Geometry check sheet. Reference: the model listing, model coordinates, mm. A direction names the side the tool comes from. Give positions to 0.01 mm unless a question says otherwise; leave off trailing zeros. Order: outer loops, then holes, each group sorted by start corner. A loop starts at its lowest first (then second) coordinate and runs counter-clockwise, first axis right, second up. Notation, with made-up numbers: M 73.25,65 L 112.25,65 A19 ccw 112.25,77 Z; hole C 32.5,15 d11. An arc over 180 degrees is marked long. Answer as CSV lines item,"result".
Autodesk Inventor part; units mm, degrees
ref_plane "Work Plane1" through (25.25, 10.625, -39.4) normal (1, 0, 0) x (0, 1, 0)
ref_plane "YZ Plane" through (0, 0, 0) normal (1, 0, 0) x (0, 1, 0)
ref_plane "XZ Plane" through (0, 0, 0) normal (0, 1, 0) x (-1, 0, 0)
sketch "Sketch2" plane through (0, 0, 0) normal (0, 1, 0) x (-1, 0, 0)
  line L0 (0, 0) -> (-20, 0)
  line L1 (-20, 0) -> (-20, -66)
  line L2 (-20, -66) -> (0, -66)
  line L3 (0, -66) -> (0, 0)
  dimension "d0" = 20
  dimension "d1" = 66
extrude "Extrusion1" add sketch "Sketch2" along normal blind 30.5
sketch "Sketch3" plane through (20, 0, 0) normal (1, 0, 0) x (0, 0, -1)
  line L0 (39.4, 20.369) -> (34.4, 20.369)
  line L1 (39.4, 10.125) -> (34.4, 10.125)
  line L2 (34.4, 18.9168) -> (34.4, 10.625)
  line L3 (34.4, 20.369) -> (34.4, 18.9308)
  line L4 (0, 0) -> (0, 30.5)
  line L5 (34.4, 20.369) -> (0, 20.369)
  line L6 (0, 20.369) -> (0, 10.125)
  line L7 (0, 10.125) -> (34.4, 10.125)
  line L8 (34.4, 10.125) -> (34.4, 20.369)
ref_plane "Work Plane1" through (25.25, 10.625, -39.4) normal (1, 0, 0) x (0, 1, 0)
extrude "Extrusion2" add sketch "Sketch3" along normal up to surface (5.25 mm away)
properties part number "lipo3s650"
(1) Section check A-A on y = 12.5. Enter the section's corners in (x, z).
The answers:
outline,"M 0,-66 L 20,-66 L 20,-34.4 L 25.25,-34.4 L 25.25,0 L 0,0 Z"
(2) Section check D-D on y = 8. Enter the section's corners in (x, z).
The answers:
outline,"M 0,-66 L 20,-66 L 20,0 L 0,0 Z"
(3) Draft check along Z on faces 1 (the face through (10, 15, 0)), 2 (the face through (23, 15, -34.4)), 3 (the face through (23, 20.369, -17)). Enter one of: +Z half, -Z half, draft (parallel to the pull), parting line (faces both ways), or undercut.
The answers:
face 1,"+Z half"
face 2,"-Z half"
face 3,"draft"
(4) Tool access check on faces 4 (the face through (23, 10.125, -17)), 5 (the face through (10, 30.5, -33)). Record the directions out of +Z, -Z, +X, -X, +Y, -Y that give a thin tool (end or side, any length) a straight path to the whole face; none if there is none.
The answers:
face 4,"+Z, -Z, +X, -Y"
face 5,"+Z, -Z, +X, -X, +Y"
(5) Section check C-C on x = 22.25. Enter the section's corners in (y, z) (3 decimals).
The answers:
outline,"M 10.125,-34.4 L 20.369,-34.4 L 20.369,0 L 10.125,0 Z"
(6) Material ranges on line 1 (X direction, y = 8, z = -24); line 2 (Y direction, x = 20.75, z = -6.5) (3 decimals), recorded low to high.
The answers:
line 1,"x = 0 to 20"
line 2,"y = 10.125 to 20.369"
(7) Gauge pin test, flat ends, axial feed: P1, Ø1.6, axis at x = 23.5, y = 16, coming from the -Z side; P2, Ø1.6, axis at x = 22.5, z = -15, coming from the -Y side (3 decimals); P3, Ø4, axis at y = 23, z = -38.5, coming from the +X side. Record the tip position at first contact, or that the pin passes through.
The answers:
P1,"stops at z = -34.4"
P2,"stops at y = 10.125"
P3,"stops at x = 20"
(8) Section check B-B on z = -20. Enter the section's corners in (x, y) (3 decimals), then the cut area to 3 significant figures.
The answers:
outline,"M 0,0 L 20,0 L 20,10.125 L 25.25,10.125 L 25.25,20.369 L 20,20.369 L 20,30.5 L 0,30.5 Z"
area,"664 mm2"
